Geometry: final body of the model. Coordinates: model frame, mm. A direction names the side the tool comes from. Coordinates: 2 decimals unless noted, no trailing zeros. Write each loop counter-clockwise with the first axis right and the second up, starting at its lowest first coordinate (ties: lowest second). Pieces come first, ordered by that corner, then holes. Notation, with made-up numbers: (83.5, 85) -> (127.5, 85) arc R19 cw to (127.5, 116) -> close; hole circle Ø5 at (72.5, 29.5). An arc over 180 degrees is marked (long way). Answer as a JSON object with one key per item and string values. Group by question number.
```python
from build123d import *

# Parameters (mm, degrees)
BOX331_W                    = 28.8
BOX331_H                    = 43.38
BOX331_DEPTH                = 20
BOX325_W                    = 56.5
BOX325_H                    = 56.5
BOX325_DEPTH                = 40
BOX327_W                    = 65
BOX327_H                    = 68
BOX327_DEPTH                = 9
COMPOUND928_ROLL_ANGLE      = 180
COMPOUND928_PLACEMENT_ANGLE = -90
CHAMFER013_SIZE             = 2


with BuildPart() as krychle331:
    # Box331 → Box331 (new body)
    with BuildSketch(Plane(origin=(-14.4, -8, 34), x_dir=(1, 0, 0), z_dir=(0, 0, 1))):
        with Locations((14.4, 21.69)):
            Rectangle(BOX331_W, BOX331_H)
    extrude(amount=BOX331_DEPTH)


with BuildPart() as krychle325:
    # Box325 → Box325 (new body)
    with BuildSketch(Plane(origin=(-28.25, -28.25, 32), x_dir=(1, 0, 0), z_dir=(0, 0, 1))):
        with Locations((28.25, 28.25)):
            Rectangle(BOX325_W, BOX325_H)
    extrude(amount=BOX325_DEPTH)


with BuildPart() as chamfer013:
    # Box327 → Box327 (new body)
    with BuildSketch(Plane(origin=(-33, -34, 32), x_dir=(1, 0, 0), z_dir=(0, 0, 1))):
        with Locations((32.5, 34)):
            Rectangle(BOX327_W, BOX327_H)
    extrude(amount=BOX327_DEPTH)

    # Cut313: cut Krychle325
    add(krychle325.part, mode=Mode.SUBTRACT)

    # Cut316: cut Krychle331
    add(krychle331.part, mode=Mode.SUBTRACT)


with BuildPart() as chamfer013_1:
    # Cut316 placement: moved
    add(chamfer013.part.moved(Location((-29, 18, 30))))


with BuildPart() as chamfer013_2:
    # Compound928 roll: moved
    add(chamfer013_1.part.rotate(Axis((0, 0, 0), (1, 0, 0)), COMPOUND928_ROLL_ANGLE))


with BuildPart() as chamfer013_3:
    # Compound928 placement: moved
    add(chamfer013_2.part.moved(Location((18, -29, 32))).rotate(Axis((18, -29, 32), (0, 0, 1)), COMPOUND928_PLACEMENT_ANGLE))

    # Chamfer013
    chamfer013_edges = [chamfer013_3.edges().sort_by_distance(p)[0] for p in [
        (0, 33, -39),
        (34, 0.5, -39),
        (-34, 23.7, -39),
        (-34, -23.2, -39),
        (0, -32, -39),
    ]]
    chamfer(chamfer013_edges, length=CHAMFER013_SIZE)


solid = chamfer013_3.part
```
Item 1: Contact query for flat-ended pins moving along their axis: pin 1 (5 mm diameter, centred on y = 13, z = -34.5, fed in from -X); pin 2 (8 mm diameter, centred on x = -22, y = -0.5, fed in from -Z); pin 3 (4.5 mm diameter, centred on x = -31.5, y = -5.5, fed in from -Z). Output: stop coordinate, or through.
Item 2: Section C-C on x = 27. Output: boundary loops of the cut face in (y, z).
Item 3: Section B-B on z = -34.5. Output: boundary loops of the cut face in (x, y).
Item 4: Section D-D on z = -31. Output: boundary loops of the cut face in (x, y), then the cut area to 3 significant figures.
Item 5: Set-up query: faces 1 (the flat face through (0, -28.25, -34)), 2 (the flat face through (-31, 0, -32)), 3 (the flat face through (2, 30, -30)). Return all of +Z, -Z, +X, -X, +Y, -Y with unobstructed straight access to the full face (end or side cutting, diameter ignored); none if empty.
Item 6: Ray query, L1, parallel to X at y = 18.5, z = -33; L2, parallel to Y at x = -10, z = -36.5. Return the intervals inside material, ascending. Write a range as [from, to].
Item 7: Mould query, pull axis Y, two halves, no side actions, for faces 4 (the flat face through (-31, -14.4, -35)), 5 (the flat face through (31, 3, -39)), 6 (the flat face through (0, -31, -38)). Classes: +Y half, -Y half, draft (parallel to the pull), parting line (faces both ways), or undercut.
Item 8: Section A-A on y = -2.5. Output: boundary loops of the cut face in (x, z).
Answer sheet:
{
 "1": {"pin 1": "stops at x = -34", "pin 2": "passes through", "pin 3": "stops at z = -32"},
 "2": {"outline": "(-32, -37) -> (-30, -39) -> (-28.25, -39) -> (-28.25, -30) -> (-32, -30) -> close; (28.25, -39) -> (31, -39) -> (33, -37) -> (33, -30) -> (28.25, -30) -> close"},
 "3": {"outline": "(-34, -32) -> (34, -32) -> (34, 33) -> (-34, 33) -> (-34, 14.4) -> (-28.25, 14.4) -> (-28.25, 28.25) -> (28.25, 28.25) -> (28.25, -28.25) -> (-28.25, -28.25) -> (-28.25, -14.4) -> (-34, -14.4) -> close"},
 "4": {"outline": "(-34, -32) -> (34, -32) -> (34, 33) -> (-34, 33) -> close; hole (-28.25, -28.25) -> (28.25, -28.25) -> (28.25, 28.25) -> (-28.25, 28.25) -> close", "area": "1,230 mm^2"},
 "5": {"face 1": "+Z, -Z", "face 2": "-Z, -X", "face 3": "+Z, +X, -X, +Y, -Y"},
 "6": {"L1": "x = [-34, -28.25], [28.25, 34]", "L2": "y = [-32, -28.25], [28.25, 33]"},
 "7": {"face 4": "undercut", "face 5": "draft", "face 6": "-Y half"},
 "8": {"outline": "(-34, -32) -> (-28.25, -32) -> (-28.25, -30) -> (-34, -30) -> close; (28.25, -39) -> (32, -39) -> (34, -37) -> (34, -30) -> (28.25, -30) -> close"}
}
